Geometry check sheet. Reference: the model listing, model coordinates, mm. A direction names the side the tool comes from. Round coordinates to 2 decimals unless told otherwise and drop trailing zeros. Order: outer loops, then holes, each group sorted by start corner. A loop starts at its lowest first (then second) coordinate and runs counter-clockwise, first axis right, second up. Notation, with made-up numbers: (-3.5, 30) - (24.5, 30) arc R31 cw to (24.5, 68) - close; hole circle Ø9 at (11, 49.25). An arc over 180 degrees is marked (long way). Use a Markdown table: item, result. Add a question column.
(1) Access from +Z, -Z, +X, -X, +Y, -Y to the whole of each face (thin tool, end or side, straight path). Record for faces 4 (the face through (2.45, -4, 11)), 5 (the face through (0, -3, 7.75)), 6 (the face through (0.323, 1.36, 3.944)), 7 (the face through (-2.685, 2.84, 8.097)).
(2) Section check D-D on z = 10.45. Record the boundary of the cut face in (x, y), then the cut area to 3 significant figures.
(3) Section check B-B on z = 6.25. Record the boundary of the cut face in (x, y).
(4) Section check C-C on x = 0.75. Record the boundary of the cut face in (y, z), then the cut area to 3 significant figures.
(5) Mould release check, pull along X, two halves, no side actions. Record for faces 1 (the face through (-4.45, 2, 9)), 2 (the face through (0, 0, 9)), 3 (the face through (0, 0.6, 12)): released by +X, released by -X, zero draft, split by the parting line, or undercut.
(6) Section check A-A on y = 1.5. Record the boundary of the cut face in (x, z), then the cut area to 3 significant figures.
(7) Gauge pin test, flat ends, axial feed: P1, Ø1, axis at x = 0.5, z = 12.5, coming from the +Y side; P2, Ø2.5, axis at x = -1, y = -3, coming from the +Z side; P3, Ø0.8, axis at y = -2, z = 6.5, coming from the +X side. Record the tip position at first contact, or that the pin passes through.
(8) Thickness scan on line 1 along Z through (x, y) = (0, 1); line 2 along Z through (x, y) = (0.5, -3.25); line 3 along X through (y, z) = (1.35, 12.45). Record the ranges inside material, lowest first. Write a range as [from, to].
Autodesk Inventor part; units mm, degrees
ref_plane "YZ Plane" through (0, 0, 0) normal (1, 0, 0) x (0, 1, 0)
ref_plane "XZ Plane" through (0, 0, 0) normal (0, 1, 0) x (-1, 0, 0)
ref_plane "XY Plane" through (0, 0, 0) normal (0, 0, 1) x (1, 0, 0)
sketch "Sketch1" plane through (0, 0, 0) normal (0, 1, 0) x (-1, 0, 0)
  circle A0 centre (0, 0) radius 1.75
  circle A1 centre (0, 0) radius 2.45
  line L0 (0.95, 1.4697) -> (0.95, -1.4697)
  line L1 (1.5, 13) -> (-1.5, 13) construction
  line L2 (-1.5, 13) -> (-1.5, 5) construction
  line L3 (-1.5, 5) -> (1.5, 5) construction
  line L4 (1.5, 5) -> (1.5, 13) construction
  line L5 (0, 5) -> (0, 0) construction
  line L6 (2.45, 0) -> (2.45, 15)
  line L7 (2.45, 15) -> (-2.45, 15)
  line L8 (-2.45, 15) -> (-2.45, 0)
  line L9 (2.45, 0) -> (2.45, -2)
  line L10 (0.45, -4) -> (-0.45, -4)
  line L11 (-2.45, -2) -> (-2.45, 0)
  arc A2 (0.45, -4) -> (2.45, -2) centre (0.45, -2) ccw
  arc A3 (-2.45, -2) -> (-0.45, -4) centre (-0.45, -2) ccw
  line L12 (2.45, 3) -> (-2.45, 3)
  dimension "d0" = 3.5
  dimension "d1" = 4.9
  dimension "d3" = 3
  dimension "d4" = 8
  dimension "d5" = 5
  dimension "d6" = 2
  dimension "d15" = 2.7
  dimension "d24" = 4
  dimension "d25" = 2
  dimension "d28" = 2
extrude "Extrusion1" add sketch "Sketch1" along normal blind 2.1 contours L12 L8 L7 L6
sketch "Sketch2" plane through (0, 0, 0) normal (0, -1, 0) x (1, 0, 0)
  line L0 (2.45, 12.8) -> (-2.45, 12.8)
  line L1 (-2.45, 12.8) -> (-2.45, 5.2)
  line L2 (-2.45, 5.2) -> (2.45, 5.2)
  line L3 (2.45, 5.2) -> (2.45, 12.8)
  line L4 (0, 0) -> (0, 5.2) construction
  line L5 (2.45, 9) -> (-2.45, 9) construction
  line L6 (-2.45, 15) -> (2.45, 15)
  line L7 (2.45, 15) -> (2.45, 3)
  dimension "d10" = 7.6
extrude "Extrusion2" add sketch "Sketch2" along normal blind 7
sketch "Sketch3" plane through (2.45, 0, -3) normal (1, 0, 0) x (0, 0, -1)
  line L0 (-15.8, 0) -> (-15.8, -7)
  line L1 (-15.8, -4) -> (-14.0679, -7)
  line L2 (-13.25, -7) -> (-13.25, 0)
  line L3 (-13.25, 0) -> (-10.75, 0)
  line L4 (-10.75, 0) -> (-10.75, -7)
  line L5 (-10.75, -7) -> (-9.9321, -7)
  line L6 (-9.9321, -7) -> (-8.2, -4)
  line L7 (-8.2, -4) -> (-9.5, -4)
  line L8 (-9.5, -4) -> (-9.5, 0)
  line L9 (-8.2, 0) -> (-8.2, -7)
  line L10 (-9.5, 0) -> (-8.2, 0)
  line L11 (-13.25, -7) -> (-14.0679, -7)
  line L12 (-15.8, -4) -> (-14.5, -4)
  line L13 (-14.5, -4) -> (-14.5, 0)
  line L14 (-14.5, 0) -> (-15.8, 0)
  line L15 (-13.25, -7) -> (-12, -6.9306) construction
  line L16 (-10.75, -7) -> (-13.25, -7)
  line L17 (-8.2, -7) -> (-15.8, -7)
  line L18 (-15.8, 0) -> (-15.8, -7)
  line L19 (-15.8, -4) -> (-15.8, -7)
  line L20 (-15.8, -7) -> (-14.0679, -7)
  line L21 (-3, 0) -> (-8.2, 0)
  line L22 (-8.2, 0) -> (-8.2, -4)
  line L23 (-12, -6.9306) -> (-12, 0) construction
  line L24 (-9.5, -4) -> (-10.75, -4) construction
  line L25 (-14.5, -4) -> (-13.25, -4) construction
  line L26 (-6, 0) -> (-18, 0)
  line L27 (-17.9, 0) -> (-18, 0)
  line L28 (-18, 0) -> (-6, 0)
  line L29 (-6.1, 0) -> (-6, 0)
  point P0 (-9.9321, -7)
  point P1 (-18, 2.1)
  point P2 (-6, 2.1)
  point P3 (-18.8, 0)
  point P4 (-14.75, -6.5676)
  point P5 (-12.25, -5.8187)
  point P6 (-10.75, -7)
  dimension "d18" = 4
  dimension "d19" = 1.25
  dimension "d20" = 1.25
  dimension "d22" = 60
extrude "Extrusion5" cut sketch "Sketch3" against normal up to surface (4.9 mm away) contours L14 L13 L12 L0 | L1 L17 L0 | L3 L4 L16 L2 | L10 L9 L7 L8 | L6 L9 L17
sketch "Sketch5" plane through (0, 2.1, 0) normal (0, 1, 0) x (1, 0, 0)
  circle A0 centre (0, 0) radius 1.05
  circle A1 centre (0, 0) radius 3.45
  line L0 (2.3973, -14.1638) -> (2.9878, -1.725)
  line L1 (2.9878, -1.725) -> (2.3973, -14.1638)
  arc A2 (-2.3973, -14.1638) -> (2.3973, -14.1638) centre (0, -14.05) ccw
  line L2 (-2.3973, -14.1638) -> (-2.9878, -1.725)
  arc A3 (-2.3973, -14.1638) -> (2.3973, -14.1638) centre (0, -14.05) ccw
  circle A4 centre (0, -4.45) radius 0.25
  circle A5 centre (0, -4.45) radius 0.6 construction
  circle A6 centre (0, -6.45) radius 0.6 construction
  circle A7 centre (0, -6.45) radius 0.25
  circle A8 centre (0, -8.45) radius 0.25
  circle A9 centre (0, -8.45) radius 0.6 construction
  circle A10 centre (0, -10.45) radius 0.25
  circle A11 centre (0, -10.45) radius 0.6 construction
  circle A12 centre (0, -12.45) radius 0.25
  circle A13 centre (0, -12.45) radius 0.6 construction
  circle A14 centre (0, -14.45) radius 0.25
  circle A15 centre (0, -14.45) radius 0.6 construction
  line L3 (0, -11.65) -> (0, 0) construction
  line L4 (0, -4.45) -> (0, -6.45)
  line L5 (0, -6.45) -> (0, -8.45)
  line L6 (0, -8.45) -> (0, -10.45)
  line L7 (0, -10.45) -> (0, -12.45)
  line L8 (0, -12.45) -> (0, -14.45)
  line L9 (0, 0) -> (-2.9878, -1.725) construction
  line L10 (0, 0) -> (2.9878, -1.725) construction
  line L11 (-2.9878, -1.725) -> (0, -1.725) construction
  line L12 (2.9878, -1.725) -> (0, -1.725) construction
  line L13 (-4.45, -3) -> (4.45, -3)
  line L14 (4.45, -3) -> (4.45, -15)
  line L15 (4.45, -15) -> (-4.45, -15)
  line L16 (-4.45, -15) -> (-4.45, -3)
  line L17 (-2.45, -3) -> (-2.45, -15)
  line L18 (2.45, -15) -> (2.45, -3)
  line L19 (-2.45, -15) -> (2.45, -15)
  line L20 (2.45, -3) -> (-2.45, -3)
  point P0 (2.45, -13.0537)
  point P1 (2.204, -15)
  point P2 (-2.204, -15)
  point P3 (-2.45, -13.0537)
  point P4 (-2.9273, -3)
  point P5 (2.9273, -3)
  dimension "d34" = 2.1
  dimension "d35" = 6.9
  dimension "d36" = 2
  dimension "d37" = 0.5
  dimension "d38" = 2.4
  dimension "d39" = 0.4
  dimension "d41" = 60
  dimension "d42" = 4.45
  dimension "d43" = 2
  dimension "d44" = 2
  dimension "d49" = 1.2
extrude "Extrusion6" add sketch "Sketch5" along normal blind 1.5 and the other way blind 2.1 contours L2 L17 L15 L16 L13 | L13 L14 L15 L18 L0
sketch "Sketch7" plane through (0, 2.1, 0) normal (0, 1, 0) x (1, 0, 0)
  line L0 (-2.9273, -3) -> (-4.45, -3)
  line L1 (4.45, -15) -> (4.45, -3)
  line L2 (-4.45, -3) -> (4.45, -3)
  line L3 (4.45, -3) -> (4.45, -15)
  line L4 (4.45, -15) -> (-4.45, -15)
  line L5 (-4.45, -15) -> (-4.45, -3)
  point P0 (0, 0)
  point P1 (4.45, -3)
extrude "Extrusion8" add sketch "Sketch7" against normal blind 2.1
sketch "Sketch6" plane through (0, 2.1, 0) normal (0, 1, 0) x (1, 0, 0)
  circle A0 centre (0, 0) radius 1.05
  circle A1 centre (0, 0) radius 3.45
  circle A2 centre (0, -14.45) radius 0.6
  circle A3 centre (0, -14.45) radius 0.6 construction
  arc A4 (-1.997, -14.1591) -> (1.997, -14.1591) centre (0, -14.05) ccw
  arc A5 (-1.997, -14.1591) -> (1.997, -14.1591) centre (0, -14.05) ccw
  circle A6 centre (0, -4.45) radius 0.6
  circle A7 centre (0, -4.45) radius 0.6 construction
  circle A8 centre (0, -6.45) radius 0.6
  circle A9 centre (0, -8.45) radius 0.6
  circle A10 centre (0, -8.45) radius 0.6 construction
  line L0 (1.997, -14.1591) -> (2.65, -2.2091)
  line L1 (2.65, -2.2091) -> (1.997, -14.1591)
  line L2 (-1.997, -14.1591) -> (-2.65, -2.2091)
  circle A11 centre (0, -10.45) radius 0.6
  circle A12 centre (0, -10.45) radius 0.6 construction
  circle A13 centre (0, -12.45) radius 0.6
  circle A14 centre (0, -12.45) radius 0.6 construction
  circle A15 centre (0, -6.45) radius 0.6 construction
  line L3 (0, -12.05) -> (0, 0) construction
  line L4 (0, -4.45) -> (0, -6.45)
  line L5 (0, -6.45) -> (0, -8.45)
  line L6 (0, -8.45) -> (0, -10.45)
  line L7 (0, -10.45) -> (0, -12.45)
  line L8 (0, -12.45) -> (0, -14.45)
  line L9 (0, 0) -> (-2.65, -2.2091) construction
  line L10 (0, 0) -> (2.65, -2.2091) construction
  line L11 (-2.65, -2.2091) -> (0, -2.2091) construction
  line L12 (2.65, -2.2091) -> (0, -2.2091) construction
  line L13 (-4.45, -3) -> (4.45, -3)
  line L14 (4.45, -3) -> (4.45, -15)
  line L15 (4.45, -15) -> (-4.45, -15)
  line L16 (-4.45, -15) -> (-4.45, -3)
  line L17 (-2.45, -3) -> (-2.45, -15)
  line L18 (2.45, -15) -> (2.45, -3)
  line L19 (-2.45, -15) -> (2.45, -15)
  line L20 (2.45, -3) -> (-2.45, -3)
  point P0 (-0.2398, -15)
  point P1 (0.2398, -15)
  dimension "d50" = 2.1
  dimension "d51" = 6.9
  dimension "d52" = 2
  dimension "d53" = 1.2
  dimension "d54" = 2
  dimension "d55" = 0.4
  dimension "d56" = 50.185
  dimension "d57" = 4.45
  dimension "d58" = 2
  dimension "d59" = 2
  dimension "d60" = 1.2
extrude "Extrusion7" cut sketch "Sketch6" against normal blind 1.5 contours A6 | A8 L4 L5 | L5 L4 A8 | A9 L5 L6 | L6 L5 A9 | A11 L6 L7 | L7 L6 A11 | A13 L7 L8 | L8 L7 A13
properties part number "PlugConnectionBigServo"
Check sheet entries:
| question | item | result |
|---|---|---|
| 1 | face 4 | +Z, -Z, +X, -Y |
| 1 | face 5 | +X, -X, -Y |
| 1 | face 6 | +Y |
| 1 | face 7 | -Z, +Y |
| 2 | outline | (-4.45, 0) - (-2.45, 0) - (-2.45, -7) - (2.45, -7) - (2.45, 0) - (4.45, 0) - (4.45, 3.6) - (2.57, 3.6) - (2.57, 2.1) - (0.6, 2.1) - (0.6, 0.6) - (-0.6, 0.6) - (-0.6, 2.1) - (-2.57, 2.1) - (-2.57, 3.6) - (-4.45, 3.6) - close |
| 2 | area | 56.8 mm2 |
| 3 | outline | (-4.45, 0) - (4.45, 0) - (4.45, 3.6) - (2.77, 3.6) - (2.77, 2.1) - (0.57, 2.1) - (0.57, 0.6) - (-0.57, 0.6) - (-0.57, 2.1) - (-2.77, 2.1) - (-2.77, 3.6) - (-4.45, 3.6) - close; (-2.45, -5.82) - (2.45, -5.82) - (2.45, -4) - (-2.45, -4) - close |
| 4 | outline | (-7, 6.93) - (-4, 5.2) - (-4, 6.5) - (0, 6.5) - (0, 3) - (2.1, 3) - (2.1, 15) - (0, 15) - (0, 11.5) - (-4, 11.5) - (-4, 12.8) - (-7, 11.07) - (-7, 10.25) - (0, 10.25) - (0, 7.75) - (-7, 7.75) - close |
| 4 | area | 45.3 mm2 |
| 5 | face 1 | released by -X |
| 5 | face 2 | zero draft |
| 5 | face 3 | undercut |
| 6 | outline | (-4.45, 3) - (4.45, 3) - (4.45, 15) - (-4.45, 15) - close; hole circle Ø1.2 at (0, 4.45); hole circle Ø1.2 at (0, 6.45); hole circle Ø1.2 at (0, 8.45); hole circle Ø1.2 at (0, 10.45); hole circle Ø1.2 at (0, 12.45) |
| 6 | area | 101 mm2 |
| 7 | P1 | stops at y = 2.1 |
| 7 | P2 | stops at z = 12.8 |
| 7 | P3 | stops at x = 2.45 |
| 8 | line 1 | z = [3, 3.85], [5.05, 5.85], [7.05, 7.85], [9.05, 9.85], [11.05, 11.85], [13.05, 15] |
| 8 | line 2 | z = [6.5, 7.75], [10.25, 11.5] |
| 8 | line 3 | x = [-4.45, -0.6], [0.6, 4.45] |
